Model file for the job. Use its own axes, mm. A direction names the side the tool comes from. Give positions to 0.01 mm unless a question says otherwise; leave off trailing zeros. Order: outer loops, then holes, each group sorted by start corner. A loop starts at its lowest first (then second) coordinate and runs counter-clockwise, first axis right, second up. Notation, with made-up numbers: M -16.75,-33 L 26.25,-33 A19 ccw 26.25,-27 Z; hole C 34,49.5 d7. An arc over 180 degrees is marked long. Return JSON: item names as keys, results as strings. Group by question number.
1. Two-plate mould, pull along X, no slides. Class faces 4 (the face through (1.216, 3.944, -1.115)), 5 (the face through (-5, 4, 4)), 6 (the face through (0, 8, 13)), 7 (the face through (0, 4, -5)): released by +X, released by -X, zero draft, split by the parting line, or undercut.
2. Slice it at C-C on z = 6.5. List the corners of the cut face in (x, y), then the cut area to 3 significant figures.
3. Slice it at D-D on x = 14. List the corners of the cut face in (y, z), then the cut area to 3 significant figures.
4. Pin check, flat tips, straight feed: pin 1 (3 mm diameter, centred on x = 7.5, y = 2.5, fed in from -Z); pin 2 (4 mm diameter, centred on y = 4.5, z = 3.5, fed in from -X). Stop position of each tip, or through.
5. Wall check: probe 1 along Z at (x, y) = (0, 6); probe 2 along X at (y, z) = (2, 1.5); probe 3 along Z at (x, y) = (9, 0.75). Give the ranges that are in metal, low to high. Write a range as [from, to].
6. Slice it at A-A on x = 0. List the corners of the cut face in (y, z), then the cut area to 3 significant figures.
7. Slice it at B-B on y = 5. List the corners of the cut face in (x, z), then the cut area to 3 significant figures.
8. 3-axis set-ups, long thin cutter, end or side, ignore diameter. For faces 1 (the face through (15, 4, 8)), 2 (the face through (0, 0, 13)), 3 (the face through (-15, 4, 8)): which of +Z, -Z, +X, -X, +Y, -Y reach the whole face in a straight line?
Autodesk Inventor part; units mm, degrees
ref_plane "YZ Plane" through (0, 0, 0) normal (1, 0, 0) x (0, 1, 0)
ref_plane "XZ Plane" through (0, 0, 0) normal (0, 1, 0) x (-1, 0, 0)
ref_plane "XY Plane" through (0, 0, 0) normal (0, 0, 1) x (1, 0, 0)
sketch "Sketch1" plane through (0, 0, 0) normal (0, 1, 0) x (-1, 0, 0)
  circle A0 centre (0, 0) radius 1.65
  line L0 (5, -5) -> (-5, -5)
  line L1 (-5, -5) -> (-5, 20)
  line L2 (-5, 20) -> (5, 20)
  line L3 (5, 20) -> (5, -5)
  circle A1 centre (0, 0) radius 5
  line L4 (25, 8) -> (-25, 8)
  line L5 (-25, 8) -> (-25, 20)
  line L6 (-25, 20) -> (25, 20)
  line L7 (25, 20) -> (25, 8)
  point P0 (-5, 0)
  point P1 (5, 0)
  point P2 (5, 8)
  point P3 (-5, 8)
  dimension "d0" = 3.3
  dimension "d1" = 10
  dimension "d2" = 20
  dimension "d5" = 12
  dimension "d6" = 20
  dimension "d7" = 20
extrude "Extrusion1" add sketch "Sketch1" along normal blind 8 contours A1 | A1 L1 L4 L3 | L4 L1 L2 L3 | L3 L6 L7 L4 | L4 L5 L6 L1
properties part number "Fix_pin"
Result:
{
 "1": {"face 4": "undercut", "face 5": "released by -X", "face 6": "zero draft", "face 7": "split by the parting line"},
 "2": {"outline": "M -5,0 L 5,0 L 5,8 L -5,8 Z", "area": "80.0 mm2"},
 "3": {"outline": "M 0,8 L 8,8 L 8,20 L 0,20 Z", "area": "96.0 mm2"},
 "4": {"pin 1": "stops at z = 8", "pin 2": "stops at x = -5"},
 "5": {"probe 1": "z = [-5, -1.65], [1.65, 20]", "probe 2": "x = [-5, -0.69], [0.69, 5]", "probe 3": "z = [8, 20]"},
 "6": {"outline": "M 0,-5 L 8,-5 L 8,-1.65 L 0,-1.65 Z; M 0,1.65 L 8,1.65 L 8,20 L 0,20 Z", "area": "174 mm2"},
 "7": {"outline": "M -25,8 L -5,8 L -5,0 A5 ccw 5,0 L 5,8 L 25,8 L 25,20 L -25,20 Z; hole C 0,0 d3.3", "area": "711 mm2"},
 "8": {"face 1": "-Z, +X, +Y, -Y", "face 2": "+Z, -Z, +X, -X, -Y", "face 3": "-Z, -X, +Y, -Y"}
}
